For this review, take the finished solid that the model builds, in its own axes (mm). A direction names the side the tool comes from. Coordinates: 2 decimals unless noted, no trailing zeros. Write each loop counter-clockwise with the first axis right and the second up, starting at its lowest first coordinate (ties: lowest second). Pieces come first, ordered by that corner, then holes.
1) Insertion check: P1, Ø1.9, axis at x = -15.5, y = -3, coming from the +Z side; P2, Ø6.5, axis at y = -4.5, z = -162.5, coming from the -X side; P3, Ø4, axis at x = -49, z = 134.5, coming from the +Y side; P4, Ø6.5, axis at x = -105, y = -5, coming from the -Z side. Each pin has a flat end and moves straight along its axis. Give the tip position at first contact, or say it passes through.
2) For faces 1 (the face through (-72, -6, -146.05)), 2 (the face through (-2, -6.35, 165)), 3 (the face through (-2, -12.7, 2)), list the 3-axis set-ups (+Z, -Z, +X, -X, +Y, -Y) from which the entire face can be reached by the end or side of a thin tool; tool diameter is ignored.
3) To check wall thickness, follow line 1 along Z through (x, y) = (76, -2); line 2 along Z through (x, y) = (-6.5, -9). State the ranges of each line that lie inside material, in increasing order.
4) We need section A-A on x = 35.5. Write out the cut boundary in (y, z), then the cut area to 3 significant figures.
5) We need section B-B on y = -3.75. Write out the cut boundary in (x, z) (3 decimals), then the cut area to 3 significant figures.
from build123d import *

# Parameters (mm, degrees)
F0_W     = 285.75
F0_H     = 342.9
F1_DEPTH = 12.7
F2_W     = 142.875
F2_H     = 12.7
F3_DEPTH = 25.4
F4_W     = 285.75
F4_H     = 6.35
F5_DEPTH = 12.7


with BuildPart() as f1:
    # F0 (on Front) → F1 (new body)
    with BuildSketch(Plane.XZ):
        Rectangle(F0_W, F0_H)
    extrude(amount=F1_DEPTH)

    # F2 (on face) → F3 (cut)
    with BuildSketch(Plane(origin=(0, 0, -171.45), x_dir=(1, 0, 0), z_dir=(0, 0, -1))):
        with Locations((-71.4375, 6.35)):
            Rectangle(F2_W, F2_H)
    extrude(amount=-F3_DEPTH, mode=Mode.SUBTRACT)

    # F4 (on face) → F5 (cut)
    with BuildSketch(Plane.XY.offset(171.45)):
        with Locations((0, -3.175)):
            Rectangle(F4_W, F4_H)
    extrude(amount=-F5_DEPTH, mode=Mode.SUBTRACT)


solid = f1.part
Result:
1. P1: stops at z = 158.75
1. P2: stops at x = 0
1. P3: stops at y = 0
1. P4: stops at z = -146.05
2. face 1: -Z, -X, +Y, -Y
2. face 2: +Z, +X, -X, +Y
2. face 3: +Z, -Z, +X, -X, -Y
3. line 1: z = -171.45 to 158.75
3. line 2: z = -146.05 to 171.45
4. outline: (-12.7, -171.45) - (0, -171.45) - (0, 158.75) - (-6.35, 158.75) - (-6.35, 171.45) - (-12.7, 171.45) - close
4. area: 4,270 mm2
5. outline: (-142.875, -146.05) - (0, -146.05) - (0, -171.45) - (142.875, -171.45) - (142.875, 158.75) - (-142.875, 158.75) - close
5. area: 90,700 mm2
